Geometry check sheet. Reference: the model listing, model coordinates, mm. A direction names the side the tool comes from. Coordinates: 2 decimals unless noted, no trailing zeros. Write each loop counter-clockwise with the first axis right and the second up, starting at its lowest first coordinate (ties: lowest second). Pieces come first, ordered by that corner, then holes. Notation, with made-up numbers: (22, 67) -> (66, 67) arc R25 cw to (66, 89) -> close; hole circle Ø7 at (32, -17). An arc over 180 degrees is marked (long way). Use a Markdown table: item, result.
```python
from build123d import *

# Parameters (mm, degrees)
F0_W     = 101.6
F0_H     = 25.4
F1_DEPTH = 12.7
F2_R     = 6.35
F3_DEPTH = 25.4
F4_R     = 6.35
F5_DEPTH = 38.1


with BuildPart() as f1:
    # F0 (on Top) → F1 (new body)
    with BuildSketch(Plane.XY):
        with Locations((17.584615, 12.7)):
            Rectangle(F0_W, F0_H)
    extrude(amount=-F1_DEPTH)

    # F2 (on face) → F3 (cut)
    with BuildSketch(Plane.XY):
        with BuildLine():
            ThreePointArc((55.684615, 6.35), (60.174744, 8.209872), (62.034615, 12.7))
            ThreePointArc((62.034615, 12.7), (60.174744, 17.190128), (55.684615, 19.05))
            ThreePointArc((55.684615, 19.05), (49.334615, 12.7), (55.684615, 6.35))
        make_face()
        with BuildLine():
            ThreePointArc((36.634615, 12.7), (34.774744, 17.190128), (30.284615, 19.05))
            ThreePointArc((30.284615, 19.05), (23.934615, 12.7), (30.284615, 6.35))
            ThreePointArc((30.284615, 6.35), (34.774744, 8.209872), (36.634615, 12.7))
        make_face()
        with BuildLine():
            ThreePointArc((-33.215385, 12.7), (-29.495641, 21.680256), (-20.515385, 25.4))
            Line((-20.515385, 25.4), (-33.215385, 25.4))
            Line((-33.215385, 25.4), (-33.215385, 12.7))
        make_face()
        with BuildLine():
            ThreePointArc((-20.515385, 0), (-29.495641, 3.719744), (-33.215385, 12.7))
            Line((-33.215385, 12.7), (-33.215385, 0))
            Line((-33.215385, 0), (-20.515385, 0))
        make_face()
        with BuildLine():
            Line((68.384615, 25.4), (55.684615, 25.4))
            ThreePointArc((55.684615, 25.4), (64.664872, 21.680256), (68.384615, 12.7))
            Line((68.384615, 12.7), (68.384615, 25.4))
        make_face()
        with BuildLine():
            Line((68.384615, 0), (68.384615, 12.7))
            ThreePointArc((68.384615, 12.7), (64.664872, 3.719744), (55.684615, 0))
            Line((55.684615, 0), (68.384615, 0))
        make_face()
        with BuildLine():
            ThreePointArc((55.684615, 6.35), (49.334615, 12.7), (55.684615, 19.05))
            Line((55.684615, 19.05), (30.284615, 19.05))
            ThreePointArc((30.284615, 19.05), (34.774744, 17.190128), (36.634615, 12.7))
            ThreePointArc((36.634615, 12.7), (34.774744, 8.209872), (30.284615, 6.35))
            Line((30.284615, 6.35), (55.684615, 6.35))
        make_face()
        with Locations((-20.515385, 12.7)):
            Circle(F2_R)
    extrude(amount=-F3_DEPTH, mode=Mode.SUBTRACT)

    # F4 (on face) → F5 (join)
    with BuildSketch(Plane.XY):
        with BuildLine():
            ThreePointArc((4.333231, 0), (13.313487, 3.719744), (17.033231, 12.7))
            ThreePointArc((17.033231, 12.7), (13.313487, 21.680256), (4.333231, 25.4))
            ThreePointArc((4.333231, 25.4), (-8.366769, 12.7), (4.333231, 0))
        make_face()
        with Locations((4.333231, 12.7)):
            Circle(F4_R, mode=Mode.SUBTRACT)
    extrude(amount=F5_DEPTH)


solid = f1.part
```
Item 1: Section check A-A on x = 32. Record the boundary of the cut face in (y, z), then the cut area to 3 significant figures.
Answer block:
| item | result |
|---|---|
| outline | (0, -12.7) -> (6.35, -12.7) -> (6.35, 0) -> (0, 0) -> close; (19.05, -12.7) -> (25.4, -12.7) -> (25.4, 0) -> (19.05, 0) -> close |
| area | 161 mm^2 |
Item 2: Section check B-B on z = -2. Record the boundary of the cut face in (x, y), then the cut area to 3 significant figures.
Answer block:
| item | result |
|---|---|
| outline | (-20.52, 0) -> (55.68, 0) arc R12.7 ccw to (68.38, 12.7) arc R12.7 ccw to (55.68, 25.4) -> (-20.52, 25.4) arc R12.7 ccw to start; hole circle Ø12.7 at (-20.52, 12.7); hole (30.28, 6.35) -> (55.68, 6.35) arc R6.35 ccw to (62.03, 12.7) arc R6.35 ccw to (55.68, 19.05) -> (30.28, 19.05) arc R6.35 ccw to start |
| area | 1,870 mm^2 |
Item 3: Section check D-D on x = -11. Record the boundary of the cut face in (y, z), then the cut area to 3 significant figures.
Answer block:
| item | result |
|---|---|
| outline | (0, -12.7) -> (25.4, -12.7) -> (25.4, 0) -> (0, 0) -> close |
| area | 323 mm^2 |
Item 4: Depth check by flat-ended pin: P1, Ø14.5, axis at x = -20.52, y = 12.7, coming from the +Z side; P2, Ø1.5, axis at y = 23, z = 21, coming from the +X side; P3, Ø2, axis at x = 41.5, y = 18, coming from the -Z side; P4, Ø6, axis at y = 16.5, z = 28.5, coming from the -X side. Enter the tip coordinate at first touch or a pass-through.
Answer block:
| item | result |
|---|---|
| P1 | stops at z = 0 |
| P2 | stops at x = 12.71 |
| P3 | passes through |
| P4 | stops at x = -8.34 |
Item 5: Mould release check, pull along X, two halves, no side actions. Record for faces 4 (the flat face through (17, 25.4, -6)), 5 (the cylindrical face through (23.936, 12.84, -6.261)): +X half, -X half, draft (parallel to the pull), parting line (faces both ways), or undercut.
Answer block:
| item | result |
|---|---|
| face 4 | draft |
| face 5 | undercut |
Item 6: Tool access check on faces 1 (the flat face through (4, 13, 0)), 2 (the flat face through (17, 0, -6)), 3 (the flat face through (43, 6.35, -6)). Record the directions out of +Z, -Z, +X, -X, +Y, -Y that give a thin tool (end or side, any length) a straight path to the whole face; none if there is none.
Answer block:
| item | result |
|---|---|
| face 1 | +Z |
| face 2 | +Z, -Z, +X, -X, -Y |
| face 3 | +Z, -Z |
Item 7: Section check C-C on z = 29.5. Record the boundary of the cut face in (x, y), then the cut area to 3 significant figures.
Answer block:
| item | result |
|---|---|
| outline | circle Ø25.4 at (4.33, 12.7); hole circle Ø12.7 at (4.33, 12.7) |
| area | 380 mm^2 |
Item 8: Thickness scan on L1, parallel to Z at x = -10.5, y = 21; L2, parallel to Y at x = 56, z = -2.5; L3, parallel to X at y = 11, z = 20. Record the ranges inside material, lowest first. Write a range as [from, to].
Answer block:
| item | result |
|---|---|
| L1 | z = [-12.7, 0] |
| L2 | y = [0, 6.36], [19.04, 25.4] |
| L3 | x = [-8.25, -1.78], [10.45, 16.92] |
